Geometry check sheet. Reference: the model listing, model coordinates, mm. A direction names the side the tool comes from. Round coordinates to 2 decimals unless told otherwise and drop trailing zeros. Write each loop counter-clockwise with the first axis right and the second up, starting at its lowest first coordinate (ties: lowest second). Pieces come first, ordered by that corner, then holes. Notation, with made-up numbers: (-0.75, 66.25) - (7.25, 66.25) arc R20 ccw to (7.25, 97.25) - close; hole circle Ø10 at (40.5, -31.75). An arc over 180 degrees is marked (long way). Return JSON: item names as keys, results as strings.
```python
from build123d import *

# Parameters (mm, degrees)
F0_R     = 0.8255
F1_DEPTH = 3.175
F2_DEPTH = 1.5875


with BuildPart() as f1:
    # F0 (on Front) → F1 (new body, symmetric)
    with BuildSketch(Plane.XZ):
        Polygon((-1.5875, -1.5875), (1.5875, -1.5875), (1.5875, 1.5875), (0, 1.5875), (-1.5875, 1.5875), align=None)
        with BuildLine():
            ThreePointArc((-1.5875, 3.175), (-1.1225320151, 2.0524679849), (0, 1.5875))
            ThreePointArc((0, 1.5875), (1.1225320151, 2.0524679849), (1.5875, 3.175))
            ThreePointArc((1.5875, 3.175), (1.1225320091, 4.2975320212), (-1.72e-08, 4.7625))
            ThreePointArc((-1.72e-08, 4.7625), (-1.1225320212, 4.2975320091), (-1.5875, 3.175))
        make_face()
        with Locations((0, 3.175)):
            Circle(F0_R, mode=Mode.SUBTRACT)
        with BuildLine():
            Line((0, 1.5875), (1.5875, 1.5875))
            Line((1.5875, 1.5875), (1.5875, 3.175))
            ThreePointArc((1.5875, 3.175), (1.1225320151, 2.0524679849), (0, 1.5875))
        make_face()
        with BuildLine():
            Line((-1.5875, 3.175), (-1.5875, 1.5875))
            Line((-1.5875, 1.5875), (0, 1.5875))
            ThreePointArc((0, 1.5875), (-1.1225320151, 2.0524679849), (-1.5875, 3.175))
        make_face()
    extrude(amount=F1_DEPTH, both=True)

    # F0 (on Front) → F2 (cut, symmetric)
    with BuildSketch(Plane.XZ):
        with BuildLine():
            Line((-2.54, 1.5875), (-1.5875, 1.5875))
            Line((-1.5875, 1.5875), (-1.5875, 3.175))
            ThreePointArc((-1.5875, 3.175), (-1.1225320212, 4.2975320091), (-1.72e-08, 4.7625))
            Line((-1.72e-08, 4.7625), (-2.54, 4.7625))
            Line((-2.54, 4.7625), (-2.54, 1.5875))
        make_face()
        with BuildLine():
            Line((-1.5875, 3.175), (-1.5875, 1.5875))
            Line((-1.5875, 1.5875), (0, 1.5875))
            ThreePointArc((0, 1.5875), (-1.1225320151, 2.0524679849), (-1.5875, 3.175))
        make_face()
        with BuildLine():
            ThreePointArc((-1.5875, 3.175), (-1.1225320151, 2.0524679849), (0, 1.5875))
            ThreePointArc((0, 1.5875), (1.1225320151, 2.0524679849), (1.5875, 3.175))
            ThreePointArc((1.5875, 3.175), (1.1225320091, 4.2975320212), (-1.72e-08, 4.7625))
            ThreePointArc((-1.72e-08, 4.7625), (-1.1225320212, 4.2975320091), (-1.5875, 3.175))
        make_face()
        with Locations((0, 3.175)):
            Circle(F0_R, mode=Mode.SUBTRACT)
        with Locations((0, 3.175)):
            Circle(F0_R)
        with BuildLine():
            Line((0, 1.5875), (1.5875, 1.5875))
            Line((1.5875, 1.5875), (1.5875, 3.175))
            ThreePointArc((1.5875, 3.175), (1.1225320151, 2.0524679849), (0, 1.5875))
        make_face()
    extrude(amount=F2_DEPTH, both=True, mode=Mode.SUBTRACT)


solid = f1.part
```
(1) Section check C-C, the plane y = -2. Enter the section's corners in (x, z) (1 decimal), plus the area to 3 significant figures.
Response values:
{"outline": "(-1.6, -1.6) - (1.6, -1.6) - (1.6, 3.2) arc R1.6 ccw to (-1.6, 3.2) - close; hole circle Ø1.7 at (0, 3.2)", "area": "16.9 mm^2"}
(2) Section check B-B, the plane x = 0.3. Enter the section's corners in (y, z) (1 decimal), plus the area to 3 significant figures.
Response values:
{"outline": "(-3.2, -1.6) - (3.2, -1.6) - (3.2, 2.4) - (1.6, 2.4) - (1.6, 1.6) - (-1.6, 1.6) - (-1.6, 2.4) - (-3.2, 2.4) - close; (-3.2, 3.9) - (-1.6, 3.9) - (-1.6, 4.7) - (-3.2, 4.7) - close; (1.6, 3.9) - (3.2, 3.9) - (3.2, 4.7) - (1.6, 4.7) - close", "area": "25.3 mm^2"}
(3) Release check for a two-part mould opening along Y. For faces 1 (the face through (0, 2, 4)), 2 (the face through (0, 0, 1.588)), 3 (the face through (0, 3.175, 1)) record: pulls with the +Y half, pulls with the -Y half, needs draft (parallel to the pull), parting line crosses it, or undercut.
Response values:
{"face 1": "needs draft", "face 2": "undercut", "face 3": "pulls with the +Y half"}
(4) Section check A-A, the plane z = 2. Enter the section's corners in (x, y) (1 decimal), plus the area to 3 significant figures.
Response values:
{"outline": "(-1.6, -3.2) - (1.6, -3.2) - (1.6, -1.6) - (-1.6, -1.6) - close; (-1.6, 1.6) - (1.6, 1.6) - (1.6, 3.2) - (-1.6, 3.2) - close", "area": "10.1 mm^2"}
(5) Access from +Z, -Z, +X, -X, +Y, -Y to the whole of each face (thin tool, end or side, straight path). Record for faces 4 (the face through (0, -3.175, 1)), 5 (the face through (1, 1.588, 2)).
Response values:
{"face 4": "+Z, -Z, +X, -X, -Y", "face 5": "+Z, +X, -X"}
(6) Section check D-D, the plane z = 2.75. Enter the section's corners in (x, y) (1 decimal).
Response values:
{"outline": "(-1.6, -3.2) - (-0.7, -3.2) - (-0.7, -1.6) - (-1.6, -1.6) - close; (-1.6, 1.6) - (-0.7, 1.6) - (-0.7, 3.2) - (-1.6, 3.2) - close; (0.7, -3.2) - (1.6, -3.2) - (1.6, -1.6) - (0.7, -1.6) - close; (0.7, 1.6) - (1.6, 1.6) - (1.6, 3.2) - (0.7, 3.2) - close"}
(7) Material ranges on line 1 along Z through (x, y) = (0, -2); line 2 along Y through (x, z) = (0.4, 4.5) (1 decimal); line 3 along Z through (x, y) = (1.35, 1.5), recorded low to high. Write a range as [from, to].
Response values:
{"line 1": "z = [-1.59, 2.35], [4, 4.76]", "line 2": "y = [-3.2, -1.6], [1.6, 3.2]", "line 3": "z = [-1.59, 1.59]"}
(8) Gauge pin test, flat end, axial feed: pin 1 (1.6 mm diameter, centred on x = -0.5, y = 0, fed in from +Z). Record the tip position at first contact, or that the pin passes through.
Response values:
{"pin 1": "stops at z = 1.59"}
